```python
from build123d import *

# Parameters (mm, degrees)
F0_R     = 1.5
F1_DEPTH = 7
F3_DEPTH = 3


with BuildPart() as f1:
    # F0 (on Front) → F1 (new body)
    with BuildSketch(Plane.XZ):
        Circle(F0_R)
    extrude(amount=F1_DEPTH)

    # F2 (on face) → F3 (join)
    with BuildSketch(Plane.XZ.offset(7)):
        with BuildLine():
            ThreePointArc((2.1650635095, -1.25), (2.4148145657, -0.6470476128), (2.5, 0))
            ThreePointArc((2.5, 0), (2.4148145657, 0.6470476128), (2.1650635095, 1.25))
            Line((2.1650635095, 1.25), (-2.1650635095, 1.25))
            ThreePointArc((-2.1650635095, 1.25), (-2.5, 0), (-2.1650635095, -1.25))
            Line((-2.1650635095, -1.25), (2.1650635095, -1.25))
        make_face()
        with BuildLine():
            ThreePointArc((2.1650635095, 1.25), (2.4148145657, 0.6470476128), (2.5, 0))
            ThreePointArc((2.5, 0), (2.4148145657, -0.6470476128), (2.1650635095, -1.25))
            Line((2.1650635095, -1.25), (5, -1.25))
            Line((5, -1.25), (5, 1.25))
            Line((5, 1.25), (2.1650635095, 1.25))
        make_face()
        with BuildLine():
            Line((-2.1650635095, 1.25), (2.1650635095, 1.25))
            ThreePointArc((2.1650635095, 1.25), (0, 2.5), (-2.1650635095, 1.25))
        make_face()
        with BuildLine():
            ThreePointArc((-2.1650635095, -1.25), (0, -2.5), (2.1650635095, -1.25))
            Line((2.1650635095, -1.25), (-2.1650635095, -1.25))
        make_face()
        with BuildLine():
            ThreePointArc((-2.1650635095, -1.25), (-2.5, 0), (-2.1650635095, 1.25))
            Line((-2.1650635095, 1.25), (-5, 1.25))
            Line((-5, 1.25), (-5, -1.25))
            Line((-5, -1.25), (-2.1650635095, -1.25))
        make_face()
    extrude(amount=F3_DEPTH)


solid = f1.part
```
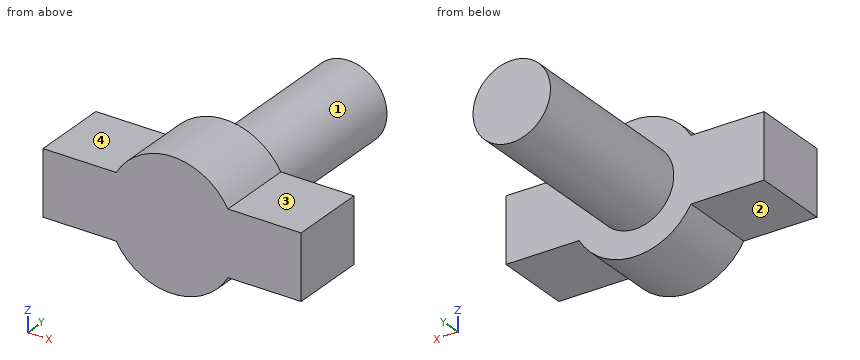
Model file for the job. Use its own axes, mm. Face numbers are marked on the shaded views. A direction names the side the tool comes from. Give positions to 0.01 mm unless a question says otherwise; leave off trailing zeros. Write each loop counter-clockwise with the first axis right and the second up, starting at its lowest first coordinate (ties: lowest second). Pieces come first, ordered by that corner, then holes. Notation, with made-up numbers: (69, 61.5) -> (96, 61.5) arc R17 cw to (96, 90.5) -> close; hole circle Ø2 at (16, 7.5). An arc over 180 degrees is marked (long way). Use CSV: the item, a comma, the result in double quotes. Start each with the question number.
1) Pin check, flat tips, straight feed: P1, Ø1.4, axis at x = -3, y = -8, coming from the +Z side; P2, Ø2.5, axis at x = -3, y = -8.5, coming from the -Z side; P3, Ø0.9, axis at x = 3, y = -8.5, coming from the -Z side; P4, Ø2, axis at x = -0.5, z = -1.5, coming from the +Y side. Stop position of each tip, or through.
2) Cut at C-C on y = -5.25. List the corners of the cut face in (x, z).
3) Cut at D-D on z = 2.05. List the corners of the cut face in (x, y).
4) Cut at A-A on y = -7.5. List the corners of the cut face in (x, z).
5) Cut at B-B on x = 0. List the corners of the cut face in (y, z), plus the area to 3 significant figures.
6) Drill centre lines: L1, parallel to Y at x = 4.5, z = 0.55; L2, parallel to Z at x = 0, y = -5.5; L3, parallel to Z at x = -4.5, y = -8.25. Where is each one in solid material? Low to high.
7) Tool access for the marked faces 1, 2, 3 and 4: list every direction of +Z, -Z, +X, -X, +Y, -Y with a clear straight run to the whole face (end or side of a thin tool).
Final values:
1,P1,"stops at z = 1.25"
1,P2,"stops at z = -1.79"
1,P3,"stops at z = -1.25"
1,P4,"stops at y = 0"
2,outline,"circle Ø3 at (0, 0)"
3,outline,"(-1.43, -10) -> (1.43, -10) -> (1.43, -7) -> (-1.43, -7) -> close"
4,outline,"(-5, -1.25) -> (-2.17, -1.25) arc R2.5 ccw to (2.17, -1.25) -> (5, -1.25) -> (5, 1.25) -> (2.17, 1.25) arc R2.5 ccw to (-2.17, 1.25) -> (-5, 1.25) -> close"
5,outline,"(-10, -2.5) -> (-7, -2.5) -> (-7, -1.5) -> (0, -1.5) -> (0, 1.5) -> (-7, 1.5) -> (-7, 2.5) -> (-10, 2.5) -> close"
5,area,"36.0 mm2"
6,L1,"y = -10 to -7"
6,L2,"z = -1.5 to 1.5"
6,L3,"z = -1.25 to 1.25"
7,face 1,"+Y"
7,face 2,"-Z, -X, +Y, -Y"
7,face 3,"+Z, +X, +Y, -Y"
7,face 4,"+Z, -X, +Y, -Y"
